Geometry: see drawing. Coordinates: mm, zero at the bounding-box minimum. Give positions to 0.01 mm unless a question says otherwise; leave off trailing zeros. Order: outer loops, then holes, each group sorted by start corner. A loop starts at its lowest first (then second) coordinate and runs counter-clockwise, first axis right, second up. Notation, with made-up numbers: M 37.25,-32.75 L 79.25,-32.75 A14 ccw 79.25,-22.75 Z; hole C 63,7 d7. An arc over 180 degrees is marked long. Use a Markdown table: item, result.
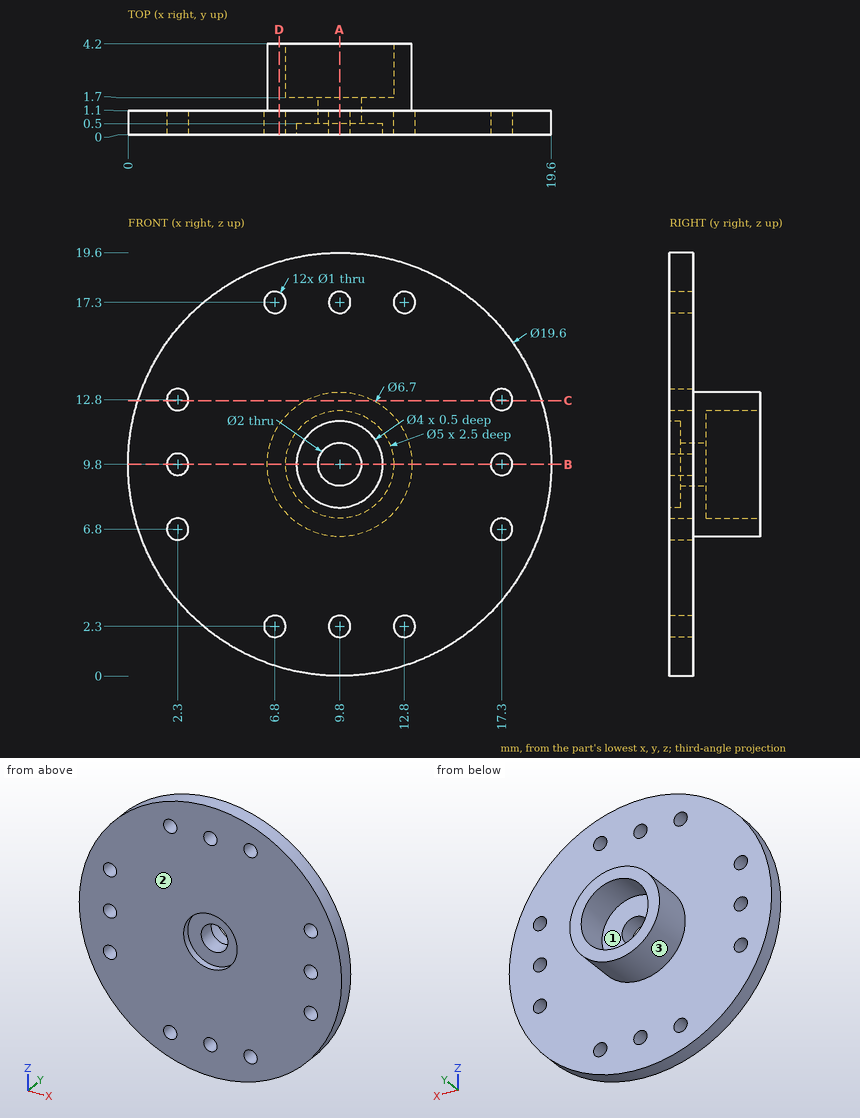
1) Mould query, pull axis Z, two halves, no side actions, for the marked faces 1, 2 and 3. Classes: released by +Z, released by -Z, zero draft, split by the parting line, or undercut.
Response values:
| item | result |
|---|---|
| face 1 | undercut |
| face 2 | zero draft |
| face 3 | split by the parting line |
2) First-contact query: pin 1 Ø8 at (x, z) = (9, 10.5) entering from +Y; pin 2 Ø1 at (y, z) = (2, 7.5) entering from +X; pin 3 Ø1.2 at (x, z) = (10, 10.5) entering from -Y; pin 4 Ø1.5 at (x, y) = (16, 2) entering from -Z. Flat tips, straight axial feed; report the tip coordinate or a pass-through.
Response values:
| item | result |
|---|---|
| pin 1 | stops at y = 4.2 |
| pin 2 | stops at x = 12.63 |
| pin 3 | stops at y = 0.5 |
| pin 4 | passes through |
3) Cut plane C-C on z = 12.75. Return loops of the section in (x, y), and give its area (3 significant figures).
Response values:
| item | result |
|---|---|
| outline | M 0.45,0 L 1.8,0 L 1.8,1.1 L 0.45,1.1 Z; M 2.8,0 L 16.8,0 L 16.8,1.1 L 11.39,1.1 L 11.39,4.2 L 8.21,4.2 L 8.21,1.1 L 2.8,1.1 Z; M 17.8,0 L 19.15,0 L 19.15,1.1 L 17.8,1.1 Z |
| area | 28.2 mm² |
4) Cut plane D-D on x = 7. Return loops of the section in (y, z), and give its area (3 significant figures).
Response values:
| item | result |
|---|---|
| outline | M 0,0.41 L 1.1,0.41 L 1.1,1.84 L 0,1.84 Z; M 0,2.76 L 1.1,2.76 L 1.1,7.96 L 4.2,7.96 L 4.2,11.64 L 1.1,11.64 L 1.1,16.84 L 0,16.84 Z; M 0,17.76 L 1.1,17.76 L 1.1,19.19 L 0,19.19 Z |
| area | 30.0 mm² |
5) Material intervals for line 1 (Z direction, x = 9.8, y = 0.9); line 2 (Z direction, x = 9.8, y = 0.4), sorted ascending. Write a range as from..to.
Response values:
| item | result |
|---|---|
| line 1 | z = 0..1.8, 2.8..8.8, 10.8..16.8, 17.8..19.6 |
| line 2 | z = 0..1.8, 2.8..7.8, 11.8..16.8, 17.8..19.6 |
6) Cut plane B-B on z = 9.8. Return loops of the section in (x, y).
Response values:
| item | result |
|---|---|
| outline | M 0,0 L 1.8,0 L 1.8,1.1 L 0,1.1 Z; M 2.8,0 L 7.8,0 L 7.8,0.5 L 8.8,0.5 L 8.8,1.7 L 7.3,1.7 L 7.3,4.2 L 6.45,4.2 L 6.45,1.1 L 2.8,1.1 Z; M 10.8,0.5 L 11.8,0.5 L 11.8,0 L 16.8,0 L 16.8,1.1 L 13.15,1.1 L 13.15,4.2 L 12.3,4.2 L 12.3,1.7 L 10.8,1.7 Z; M 17.8,0 L 19.6,0 L 19.6,1.1 L 17.8,1.1 Z |
7) Cut plane A-A on x = 9.8. Return loops of the section in (y, z), and give its area (3 significant figures).
Response values:
| item | result |
|---|---|
| outline | M 0,0 L 1.1,0 L 1.1,1.8 L 0,1.8 Z; M 0,2.8 L 1.1,2.8 L 1.1,6.45 L 4.2,6.45 L 4.2,7.3 L 1.7,7.3 L 1.7,8.8 L 0.5,8.8 L 0.5,7.8 L 0,7.8 Z; M 0,11.8 L 0.5,11.8 L 0.5,10.8 L 1.7,10.8 L 1.7,12.3 L 4.2,12.3 L 4.2,13.15 L 1.1,13.15 L 1.1,16.8 L 0,16.8 Z; M 0,17.8 L 1.1,17.8 L 1.1,19.6 L 0,19.6 Z |
| area | 23.2 mm² |
